Could you check a few things on this model? Use its own coordinates, in mm. Face numbers are marked on the shaded views. A direction names the side the tool comes from. Coordinates: 2 decimals unless noted, no trailing zeros. Loops run counter-clockwise (first coordinate to the right, second up) from the corner with the lowest first, then second, coordinate; pieces in that order, holes last. Notation, with made-up numbers: (19, 88) - (30, 88) arc R10 ccw to (30, 98) - close; hole circle Ø1 at (-38.5, 46). An arc over 180 degrees is marked (long way). One line per question, with ' | ' between items. Start each with the question number.
1. I want a section at A-A, the plane z = 0. Write out the boundary of the cut face in (x, y).
2. I want a section at B-B, the plane y = 39. Write out the boundary of the cut face in (x, z), then the cut area to 3 significant figures.
3. I'm going to push flat-ended pins straight in: P1, Ø2, axis at y = 43.5, z = -1, coming from the +X side; P2, Ø5, axis at x = -2.5, y = 23.5, coming from the +Z side; P3, Ø3, axis at x = -0.5, y = 7.5, coming from the -Z side. Where does each tip first touch, or does it pass through?
4. Which directions (+Z, -Z, +X, -X, +Y, -Y) give clear straight access to the entire face, cutting with the end or side of a thin tool? Please do the marked faces 1 and 2.
5. Please list where these lines run through material, in increasing order: L1, parallel to Y at x = 1.5, z = -2.75; L2, parallel to Z at x = -1.5, y = 22.5; L3, parallel to Y at x = 0.5, z = 0.25. Write a range as [from, to].
from build123d import *

# Parameters (mm, degrees)
SKETCH_1_R          = 4.5
EXTRUDE_1_DEPTH     = 3.5
SKETCH_2_R          = 2.5
EXTRUDE_2_DEPTH     = 55
SKETCH_3_R          = 2
EXTRUDE_3_DEPTH     = 8
CUT_EXTRUDE_1_DEPTH = 2.5
CHAMFER_1_SIZE      = 0.25


with BuildPart() as part:
    # 草图1 → 凸台-拉伸1 (new body)
    with BuildSketch(Plane(origin=(0, 0, 0), x_dir=(1, 0, 0), z_dir=(0, 1, 0))):
        with Locations(Location((0, 0, 0), (0, 0, 270))):
            Circle(SKETCH_1_R)
    extrude(amount=-EXTRUDE_1_DEPTH)

    # 草图2 → 凸台-拉伸2 (add)
    with BuildSketch(Plane(origin=(0, 0, 0), x_dir=(1, 0, 0), z_dir=(0, 1, 0))):
        with Locations(Location((0, 0, 0), (0, 0, 270))):
            Circle(SKETCH_2_R)
    extrude(amount=EXTRUDE_2_DEPTH)

    # 草图3 → 凸台-拉伸3 (add)
    with BuildSketch(Plane(origin=(0, 55, 0), x_dir=(1, 0, 0), z_dir=(0, 1, 0))):
        with Locations(Location((0, 0, 0), (0, 0, 270))):
            Circle(SKETCH_3_R)
    extrude(amount=EXTRUDE_3_DEPTH)

    # 草图4 → 切除-拉伸1 (cut)
    with BuildSketch(Plane.XZ.offset(3.5)):
        Polygon((1.5, -0.866025404), (1.5, 0.866025404), (0, 1.732050808), (-1.5, 0.866025404), (-1.5, -0.866025404), (0, -1.732050808), align=None)
    extrude(amount=-CUT_EXTRUDE_1_DEPTH, mode=Mode.SUBTRACT)

    # 倒角1
    chamfer_1_edges = [part.edges().sort_by_distance(p)[0] for p in [
        (0, 0, -4.5),
        (0, -3.5, -4.5),
    ]]
    chamfer(chamfer_1_edges, length=CHAMFER_1_SIZE)


solid = part.part
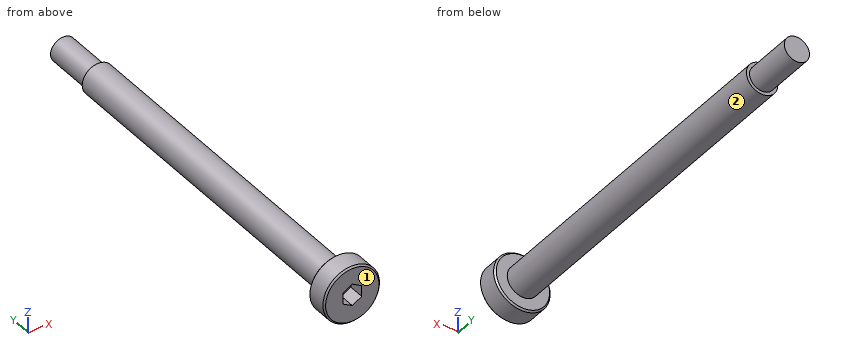
Results are:
1) outline: (-4.5, -3.25) - (-4.25, -3.5) - (-1.5, -3.5) - (-1.5, -1) - (1.5, -1) - (1.5, -3.5) - (4.25, -3.5) - (4.5, -3.25) - (4.5, -0.25) - (4.25, 0) - (2.5, 0) - (2.5, 55) - (2, 55) - (2, 63) - (-2, 63) - (-2, 55) - (-2.5, 55) - (-2.5, 0) - (-4.25, 0) - (-4.5, -0.25) - close
2) outline: circle Ø5 at (0, 0) | area: 19.6 mm2
3) P1: stops at x = 2.5 | P2: stops at z = 2.5 | P3: stops at z = -2.5
4) face 1: +Z, -Z, +X, -X, -Y | face 2: +Y
5) L1: y = [-3.5, 0] | L2: z = [-2, 2] | L3: y = [-1, 63]
